```python
from build123d import *
from OCP.BRepFilletAPI import BRepFilletAPI_MakeChamfer

# Parameters (mm, degrees)
SKETCH_1_R          = 30
EXTRUDE_1_DEPTH     = 10
SKETCH_3_R          = 4.064215012
CUT_EXTRUDE_1_DEPTH = 7
SKETCH_4_OUTSIDE_W  = 79.088
SKETCH_4_OUTSIDE_H  = 79.088
SKETCH_4_OUTSIDE_R  = 28.3
CUT_EXTRUDE_2_DEPTH = 5
CHAMFER_2_SIZE      = 1
CHAMFER_2_SIZE2     = 1.732050808


with BuildPart() as part:
    # 스케치1 → 보스-돌출1 (new body)
    with BuildSketch(Plane.XY):
        Circle(SKETCH_1_R)
        Polygon((4.5, 22.3), (2.029624384, 8), (1.014812192, 6.242293723), (-1.014812192, 6.242293723), (-2.029624384, 8), (-4.5, 22.3), (-2.25, 26.197114317), (2.25, 26.197114317), align=None, mode=Mode.SUBTRACT)
        Polygon((23.812366504, 11.15), (21.562366504, 15.047114317), (17.062366504, 15.047114317), (5.913391038, 5.757706277), (4.898578846, 4), (5.913391038, 2.242293723), (7.943015422, 2.242293723), (21.562366504, 7.252885683), align=None, mode=Mode.SUBTRACT)
        Polygon((21.562366504, -15.047114317), (23.812366504, -11.15), (21.562366504, -7.252885683), (7.943015422, -2.242293723), (5.913391038, -2.242293723), (4.898578846, -4), (5.913391038, -5.757706277), (17.062366504, -15.047114317), align=None, mode=Mode.SUBTRACT)
        Polygon((-2.25, -26.197114317), (2.25, -26.197114317), (4.5, -22.3), (2.029624384, -8), (1.014812192, -6.242293723), (-1.014812192, -6.242293723), (-2.029624384, -8), (-4.5, -22.3), align=None, mode=Mode.SUBTRACT)
        Polygon((-23.812366504, -11.15), (-21.562366504, -15.047114317), (-17.062366504, -15.047114317), (-5.913391038, -5.757706277), (-4.898578846, -4), (-5.913391038, -2.242293723), (-7.943015422, -2.242293723), (-21.562366504, -7.252885683), align=None, mode=Mode.SUBTRACT)
        Polygon((-21.562366504, 15.047114317), (-23.812366504, 11.15), (-21.562366504, 7.252885683), (-7.943015422, 2.242293723), (-5.913391038, 2.242293723), (-4.898578846, 4), (-5.913391038, 5.757706277), (-17.062366504, 15.047114317), align=None, mode=Mode.SUBTRACT)
    extrude(amount=EXTRUDE_1_DEPTH)

    # 스케치3 → 컷-돌출1 (cut)
    with BuildSketch(Plane(origin=(0, 0, 0), x_dir=(-1, 0, 0), z_dir=(0, 0, -1))):
        Circle(SKETCH_3_R)
    extrude(amount=-CUT_EXTRUDE_1_DEPTH, mode=Mode.SUBTRACT)

    # 스케치4 outside → 컷-돌출2 (cut)
    with BuildSketch(Plane(origin=(0, 0, 0), x_dir=(-1, 0, 0), z_dir=(0, 0, -1))):
        Rectangle(SKETCH_4_OUTSIDE_W, SKETCH_4_OUTSIDE_H)
        Circle(SKETCH_4_OUTSIDE_R, mode=Mode.SUBTRACT)
    extrude(amount=-CUT_EXTRUDE_2_DEPTH, mode=Mode.SUBTRACT)

    # 모따기2: one chamfer whose edges measure the first distance from different faces: ONE call of the kernel's chamfer builder (chamfer() names one face for all edges)
    chamfer_2_edges_1 = [part.edges().sort_by_distance(p)[0] for p in [
        (5.405984942, -3.121146861, 10),
        (1.522218288, -7.121146861, 10),
        (1.522218288, 7.121146861, 10),
        (3.264812192, -15.15, 10),
        (3.375, -24.248557159, 10),
        (0, -26.197114317, 10),
        (-3.375, -24.248557159, 10),
        (-3.264812192, -15.15, 10),
        (-1.522218288, -7.121146861, 10),
        (0, -6.242293723, 10),
        (-5.405984942, -4.878853139, 10),
        (-11.487878771, -10.402410297, 10),
        (-19.312366504, -15.047114317, 10),
        (0, 6.242293723, 10),
        (-22.687366504, -13.098557159, 10),
        (-22.687366504, -9.201442841, 10),
        (-14.752690963, -4.747589703, 10),
        (-6.92820323, -2.242293723, 10),
        (-5.405984942, -3.121146861, 10),
        (-6.92820323, 2.242293723, 10),
        (-14.752690963, 4.747589703, 10),
        (-22.687366504, 9.201442841, 10),
        (-22.687366504, 13.098557159, 10),
        (-19.312366504, 15.047114317, 10),
        (-1.522218288, 7.121146861, 10),
        (-11.487878771, 10.402410297, 10),
        (-5.405984942, 4.878853139, 10),
        (-5.405984942, 3.121146861, 10),
        (-3.264812192, 15.15, 10),
        (-3.375, 24.248557159, 10),
        (0, 26.197114317, 10),
        (3.375, 24.248557159, 10),
        (3.264812192, 15.15, 10),
        (5.405984942, 4.878853139, 10),
        (11.487878771, 10.402410297, 10),
        (19.312366504, 15.047114317, 10),
        (22.687366504, 13.098557159, 10),
        (22.687366504, 9.201442841, 10),
        (14.752690963, 4.747589703, 10),
        (6.92820323, 2.242293723, 10),
        (5.405984942, 3.121146861, 10),
        (6.92820323, -2.242293723, 10),
        (14.752690963, -4.747589703, 10),
        (22.687366504, -9.201442841, 10),
        (22.687366504, -13.098557159, 10),
        (19.312366504, -15.047114317, 10),
        (11.487878771, -10.402410297, 10),
        (5.405984942, -4.878853139, 10),
    ]]
    chamfer_2_side_1 = [part.faces().sort_by_distance(p)[0] for p in [
        (0, 0, 10),
    ]]
    chamfer_2_edges_2 = [part.edges().sort_by_distance(p)[0] for p in [
        (-30, 0, 10),
    ]]
    chamfer_2_side_2 = [part.faces().sort_by_distance(p)[0] for p in [
        (-30, 0, 7.5),
    ]]
    chamfer_2 = BRepFilletAPI_MakeChamfer(part.part.solid().wrapped)
    for e in chamfer_2_edges_1:
        chamfer_2.Add(CHAMFER_2_SIZE, CHAMFER_2_SIZE2, e.wrapped, chamfer_2_side_1[0].wrapped)  # the first distance lies on this face
    for e in chamfer_2_edges_2:
        chamfer_2.Add(CHAMFER_2_SIZE, CHAMFER_2_SIZE2, e.wrapped, chamfer_2_side_2[0].wrapped)  # the first distance lies on this face
    add(Compound.cast(chamfer_2.Shape()), mode=Mode.REPLACE)


solid = part.part
```
Here's how the part is built. I have some questions about the finished solid (model axes, mm). A direction names the side the tool comes from. Round coordinates to 2 decimals unless told otherwise and drop trailing zeros. Order: outer loops, then holes, each group sorted by start corner. A loop starts at its lowest first (then second) coordinate and runs counter-clockwise, first axis right, second up. Notation, with made-up numbers: M 85,61.25 L 91,61.25 A12 ccw 91,83.25 Z; hole C 62,34 d10. An arc over 180 degrees is marked long. Answer in a Markdown table with one row per item.
Item 1: Imagine slicing it at A-A, the plane x = 0. Write out the boundary of the cut face in (y, z).
A:
| item | result |
|---|---|
| outline | M -30,5 L -28.3,5 L -28.3,0 L -26.2,0 L -26.2,8.27 L -27.2,10 L -28.27,10 L -30,9 Z; M -6.24,0 L -4.06,0 L -4.06,7 L 4.06,7 L 4.06,0 L 6.24,0 L 6.24,8.27 L 5.24,10 L -5.24,10 L -6.24,8.27 Z; M 26.2,0 L 28.3,0 L 28.3,5 L 30,5 L 30,9 L 28.27,10 L 27.2,10 L 26.2,8.27 Z |
Item 2: Thinking about a two-plate mould opening in Y: for faces 3 (the face through (-19, 15.047, 4)), 4 (the face through (-11.41, 10.34, 4.08)), which applies, +Y half, -Y half, draft (parallel to the pull), parting line (faces both ways), or undercut?
A:
| item | result |
|---|---|
| face 3 | undercut |
| face 4 | undercut |
Item 3: For faces 1 (the face through (0, -26.197, 4)), 2 (the face through (3.784, -15.261, 9.122)), which set-ups out of +Z, -Z, +X, -X, +Y, -Y let a thin tool reach every point of the face, with its end or its side?
A:
| item | result |
|---|---|
| face 1 | +Z, -Z |
| face 2 | +Z |
Item 4: I'm going to push flat-ended pins straight in: pin 1 (6 mm diameter, centred on y = 19, z = 7, fed in from -X); pin 2 (1.3 mm diameter, centred on x = 20, z = 2.5, fed in from -Y); pin 3 (1.6 mm diameter, centred on x = -0.5, z = 5.5, fed in from -Y). Where does each tip first touch, or does it pass through?
A:
| item | result |
|---|---|
| pin 1 | stops at x = -25.38 |
| pin 2 | stops at y = -20.65 |
| pin 3 | stops at y = -30 |
Item 5: Imagine slicing it at B-B, the plane y = 0. Write out the boundary of the cut face in (x, z).
A:
| item | result |
|---|---|
| outline | M -30,5 L -28.3,5 L -28.3,0 L -4.06,0 L -4.06,7 L 4.06,7 L 4.06,0 L 28.3,0 L 28.3,5 L 30,5 L 30,9 L 28.27,10 L -28.27,10 L -30,9 Z |
Item 6: If I drill on L1, parallel to Y at x = 0, z = 5.5; L2, parallel to Y at x = 0, z = 3; L3, parallel to Y at x = -10, z = 6.25, over which ranges is the centre line in solid material (lowest first)? Write a range as from..to.
A:
| item | result |
|---|---|
| L1 | y = -30..-26.2, -6.24..-4.06, 4.06..6.24, 26.2..30 |
| L2 | y = -28.3..-26.2, -6.24..-4.06, 4.06..6.24, 26.2..28.3 |
| L3 | y = -28.28..-9.16, -3..3, 9.16..28.28 |
Item 7: Imagine slicing it at C-C, the plane y = 13. State how many separate pieces and enclosed holes the cut face has, and give its area (3 significant figures).
A:
| item | result |
|---|---|
| separate pieces | 4 |
| enclosed holes | 0 |
| area | 293 mm2 |
